Can you work these out from the drawing? Everything is in mm from the part's minimum corner. A direction names the side the tool comes from. Give positions to 0.01 mm unless a question says otherwise; leave off trailing zeros. Order: outer loops, then holes, each group sorted by start corner. A loop starts at its lowest first (then second) coordinate and runs counter-clockwise, first axis right, second up. Notation, with made-up numbers: M 3.25,67.5 L 20.25,67.5 A13 ccw 20.25,73.5 Z; hole C -27,28 d5. An arc over 180 degrees is marked long. Answer in a Markdown table with one row per item. Add a question column.
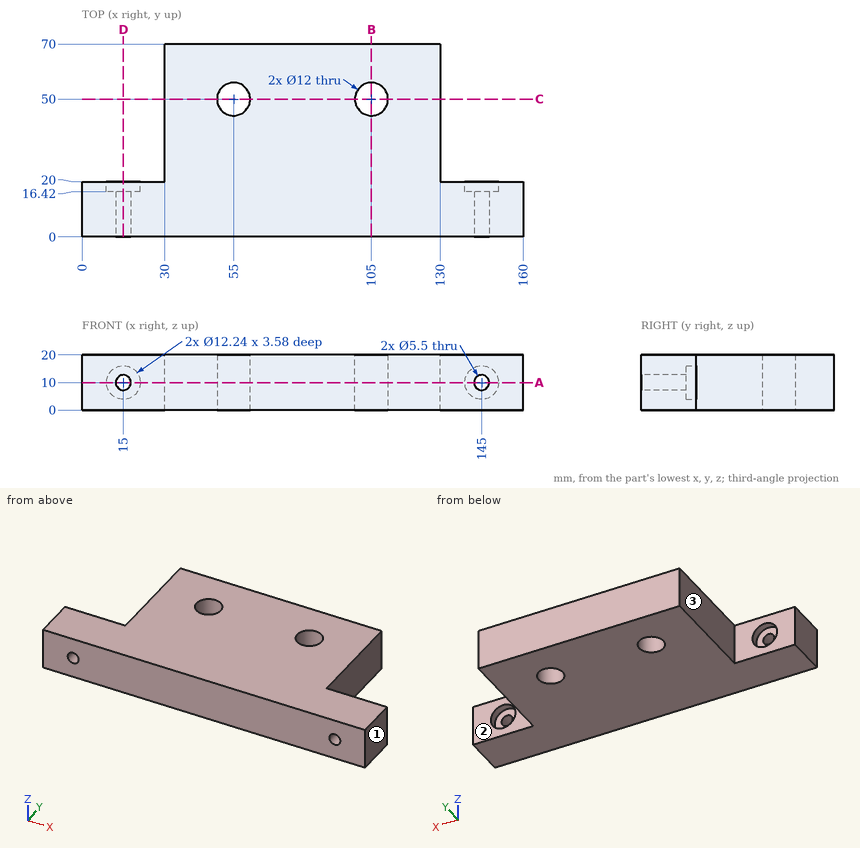
1. If I drill on line 1 along X through (y, z) = (12, 10); line 2 along Z through (x, y) = (145, 8); line 3 along X through (y, z) = (55.5, 13), over which ranges is the centre line in solid material (lowest first)? Write a range as [from, to].
2. For the marked faces 1, 2 and 3, which set-ups out of +Z, -Z, +X, -X, +Y, -Y let a thin tool reach every point of the face, with its end or its side?
3. Suppose I cut it at B-B on x = 105. List the corners of the cut face in (y, z) for me, plus the area to 3 significant figures.
4. Suppose I cut it at A-A on z = 10. List the corners of the cut face in (x, y) for me, plus the area to 3 significant figures.
5. Suppose I cut it at C-C on y = 50. List the corners of the cut face in (x, z) for me, plus the area to 3 significant figures.
6. Suppose I cut it at D-D on x = 15. List the corners of the cut face in (y, z) for me, plus the area to 3 significant figures.
7. Will these pins go through, and if not, where does the flat tip stop? P1, Ø2, axis at y = 42, z = 6, coming from the +X side; P2, Ø8, axis at x = 21.5, y = 27.5, coming from the -Z side; P3, Ø3.5, axis at x = 15.5, z = 12.5, coming from the +Y side; P4, Ø6, axis at x = 17.5, z = 12.5, coming from the +Y side.
Findings below:
| question | item | result |
|---|---|---|
| 1 | line 1 | [0, 12.25], [17.75, 142.25], [147.75, 160] |
| 1 | line 2 | [0, 7.25], [12.75, 20] |
| 1 | line 3 | [30, 52.6], [57.4, 102.6], [107.4, 130] |
| 2 | face 1 | +Z, -Z, +X, +Y, -Y |
| 2 | face 2 | +Z, -Z, +X, +Y |
| 2 | face 3 | +Z, -Z, -X, +Y |
| 3 | outline | M 0,0 L 44,0 L 44,20 L 0,20 Z; M 56,0 L 70,0 L 70,20 L 56,20 Z |
| 3 | area | 1,160 mm2 |
| 4 | outline | M 0,0 L 12.25,0 L 12.25,16.42 L 8.88,16.42 L 8.88,20 L 0,20 Z; M 17.75,0 L 142.25,0 L 142.25,16.42 L 138.88,16.42 L 138.88,20 L 130,20 L 130,70 L 30,70 L 30,20 L 21.12,20 L 21.12,16.42 L 17.75,16.42 Z; M 147.75,0 L 160,0 L 160,20 L 151.12,20 L 151.12,16.42 L 147.75,16.42 Z; hole C 55,50 d12; hole C 105,50 d12 |
| 4 | area | 7,710 mm2 |
| 5 | outline | M 30,0 L 49,0 L 49,20 L 30,20 Z; M 61,0 L 99,0 L 99,20 L 61,20 Z; M 111,0 L 130,0 L 130,20 L 111,20 Z |
| 5 | area | 1,520 mm2 |
| 6 | outline | M 0,0 L 20,0 L 20,3.88 L 16.42,3.88 L 16.42,7.25 L 0,7.25 Z; M 0,12.75 L 16.42,12.75 L 16.42,16.12 L 20,16.12 L 20,20 L 0,20 Z |
| 6 | area | 266 mm2 |
| 7 | P1 | x = 130 |
| 7 | P2 | through |
| 7 | P3 | y = 16.42 |
| 7 | P4 | y = 20 |
